The model under review builds one solid part; all positions refer to its coordinate system, in mm. A direction names the side the tool comes from. Coordinates: 2 decimals unless noted, no trailing zeros. Order: outer loops, then holes, each group sorted by start corner. A loop starts at its lowest first (then second) coordinate and runs counter-clockwise, first axis right, second up.
```python
from build123d import *

# Parameters (mm, degrees)
SKETCH_W        = 75.4
SKETCH_H        = 100
PAD_DEPTH       = 16.6
SKETCH005_W     = 71.4
SKETCH005_H     = 96
POCKET_DEPTH    = 14.6
SKETCH006_W     = 21.6
SKETCH006_H     = 11.8
POCKET001_DEPTH = 2
SKETCH007_W     = 21.6
SKETCH007_H     = 11.8
POCKET002_DEPTH = 2
SKETCH008_W     = 7.6
SKETCH008_H     = 8.2
POCKET003_DEPTH = 2
POCKET004_DEPTH = 2
SKETCH010_R     = 3.9
SKETCH010_W     = 16
SKETCH010_H     = 26.5
POCKET005_DEPTH = 2
POCKET005_TAPER = 45
SKETCH011_W     = 15
SKETCH011_H     = 2
PAD005_DEPTH    = 14.6
SKETCH012_R     = 1.1
PAD006_DEPTH    = 8.6
SKETCH013_R     = 1.1
PAD007_DEPTH    = 10.4
FILLET_R        = 2
FILLET001_R     = 4
FILLET002_R     = 1
FILLET003_R     = 6
FILLET004_R     = 5.5
FILLET005_R     = 4
SKETCH022_W     = 31.2
SKETCH022_H     = 29
SKETCH022_W_2   = 28.8
SKETCH022_H_2   = 26.6
PAD013_DEPTH    = 3.4
FILLET011_R     = 8


with BuildPart() as part:
    # Sketch → Pad (new body)
    with BuildSketch(Plane.XY):
        with Locations((0, -28.5)):
            Rectangle(SKETCH_W, SKETCH_H)
    extrude(amount=PAD_DEPTH)

    # Sketch005 (on Face5 of Pad) → Pocket (cut)
    with BuildSketch(Plane(origin=(0, 0, 0), x_dir=(1, 0, 0), z_dir=(0, 0, -1))):
        with Locations((0, 28.5)):
            Rectangle(SKETCH005_W, SKETCH005_H)
    extrude(amount=-POCKET_DEPTH, mode=Mode.SUBTRACT)

    # Sketch006 (on Face3 of Pocket) → Pocket001 (cut)
    with BuildSketch(Plane.YZ.offset(37.7)):
        with Locations((0, 5.9)):
            Rectangle(SKETCH006_W, SKETCH006_H)
    extrude(amount=-POCKET001_DEPTH, mode=Mode.SUBTRACT)

    # Sketch007 (on Face2 of Pocket) → Pocket002 (cut)
    with BuildSketch(Plane(origin=(-37.7, 0, 0), x_dir=(0, -1, 0), z_dir=(-1, 0, 0))):
        with Locations((0, 5.9)):
            Rectangle(SKETCH007_W, SKETCH007_H)
    extrude(amount=-POCKET002_DEPTH, mode=Mode.SUBTRACT)

    # Sketch008 (on Face1 of Pocket) → Pocket003 (cut)
    with BuildSketch(Plane(origin=(0, 21.5, 0), x_dir=(-1, 0, 0), z_dir=(0, 1, 0))):
        with Locations((22, 4.1)):
            Rectangle(SKETCH008_W, SKETCH008_H)
    extrude(amount=-POCKET003_DEPTH, mode=Mode.SUBTRACT)

    # Sketch009 (on Face5 of Pocket) → Pocket004 (cut)
    with BuildSketch(Plane.XY.offset(16.6)):
        with BuildLine():
            Line((15.825713, -15.337742), (15.825713, -16.321696))
            ThreePointArc((15.825713, -16.321696), (16.397859, -17.902616), (17.897046, -18.663599))
            Line((17.897046, -18.663599), (25.282393, -18.663599))
            ThreePointArc((25.282393, -18.663599), (26.185781, -18.272491), (26.544973, -17.355945))
            Line((26.544973, -14.219638), (26.544973, -17.355945))
            ThreePointArc((26.544973, -14.219638), (26.159832, -13.349897), (25.274241, -13.00275))
            Line((17.921865, -13.00275), (25.274241, -13.00275))
            ThreePointArc((17.921865, -13.00275), (16.411472, -13.755218), (15.825713, -15.337742))
        make_face()
    extrude(amount=-POCKET004_DEPTH, mode=Mode.SUBTRACT)

    # Sketch010 (on Face5 of Pocket) → Pocket005 (cut)
    with BuildSketch(Plane.XY.offset(16.6)):
        with Locations((-17.145816, -1.900756)):
            Circle(SKETCH010_R)
        with Locations((10, 2.4)):
            Rectangle(SKETCH010_W, SKETCH010_H)
    extrude(amount=-POCKET005_DEPTH, taper=POCKET005_TAPER, mode=Mode.SUBTRACT)

    # Sketch011 (on Face11 of Pocket) → Pad005 (join)
    with BuildSketch(Plane(origin=(0, 0, 14.6), x_dir=(1, 0, 0), z_dir=(0, 0, -1))):
        with Locations((-28.2, 47.5)):
            Rectangle(SKETCH011_W, SKETCH011_H)
        with Locations((-28.2, 20.5)):
            Rectangle(SKETCH011_W, SKETCH011_H)
        with Locations((28.2, 47.5)):
            Rectangle(SKETCH011_W, SKETCH011_H)
        with Locations((28.2, 20.5)):
            Rectangle(SKETCH011_W, SKETCH011_H)
    extrude(amount=PAD005_DEPTH)

    # Sketch012 (on Face11 of Pocket) → Pad006 (join)
    with BuildSketch(Plane(origin=(0, 0, 14.6), x_dir=(1, 0, 0), z_dir=(0, 0, -1))):
        with BuildLine():
            Line((-35.7, -12.5), (-31.85, -12.5))
            ThreePointArc((-28.85, -15.5), (-29.72868, -13.37868), (-31.85, -12.5))
            Line((-28.85, -19.5), (-28.85, -15.5))
            Line((-28.85, -19.5), (-35.7, -19.5))
            Line((-35.7, -12.5), (-35.7, -19.5))
        make_face()
        with Locations((-31.85, -15.5)):
            Circle(SKETCH012_R, mode=Mode.SUBTRACT)
        with BuildLine():
            Line((28.85, -19.5), (28.85, -15.5))
            ThreePointArc((31.85, -12.5), (29.72868, -13.37868), (28.85, -15.5))
            Line((35.7, -12.5), (31.85, -12.5))
            Line((35.7, -12.5), (35.7, -19.5))
            Line((28.85, -19.5), (35.7, -19.5))
        make_face()
        with Locations((31.85, -15.5)):
            Circle(SKETCH012_R, mode=Mode.SUBTRACT)
        with BuildLine():
            Line((-35.7, 12.5), (-35.7, 19.5))
            Line((-35.7, 19.5), (-28.85, 19.5))
            Line((-28.85, 19.5), (-28.85, 15.5))
            ThreePointArc((-31.85, 12.5), (-29.72868, 13.37868), (-28.85, 15.5))
            Line((-35.7, 12.5), (-31.85, 12.5))
        make_face()
        with Locations((-31.85, 15.5)):
            Circle(SKETCH012_R, mode=Mode.SUBTRACT)
        with BuildLine():
            Line((31.85, 12.5), (35.7, 12.5))
            Line((35.7, 12.5), (35.7, 19.5))
            Line((35.7, 19.5), (28.85, 19.5))
            Line((28.85, 19.5), (28.85, 15.5))
            ThreePointArc((28.85, 15.5), (29.72868, 13.37868), (31.85, 12.5))
        make_face()
        with Locations((31.85, 15.5)):
            Circle(SKETCH012_R, mode=Mode.SUBTRACT)
    extrude(amount=PAD006_DEPTH)

    # Sketch013 (on Face11 of Pocket) → Pad007 (join)
    with BuildSketch(Plane(origin=(0, 0, 14.6), x_dir=(1, 0, 0), z_dir=(0, 0, -1))):
        with BuildLine():
            Line((-35.7, 76.5), (-29.35, 76.5))
            Line((-29.35, 76.5), (-29.35, 72.5))
            ThreePointArc((-31.85, 70), (-30.082233, 70.732233), (-29.35, 72.5))
            Line((-35.7, 70), (-31.85, 70))
            Line((-35.7, 76.5), (-35.7, 70))
        make_face()
        with Locations((-31.85, 72.5)):
            Circle(SKETCH013_R, mode=Mode.SUBTRACT)
        with BuildLine():
            Line((35.7, 76.5), (35.7, 70))
            Line((35.7, 70), (31.85, 70))
            ThreePointArc((29.35, 72.5), (30.082233, 70.732233), (31.85, 70))
            Line((29.35, 76.5), (29.35, 72.5))
            Line((35.7, 76.5), (29.35, 76.5))
        make_face()
        with Locations((31.85, 72.5)):
            Circle(SKETCH013_R, mode=Mode.SUBTRACT)
    extrude(amount=PAD007_DEPTH)

    # Fillet
    fillet_edges = [part.edges().sort_by_distance(p)[0] for p in [
        (-35.7, 0, 14.6),
        (-35.7, -34, 14.6),
        (-35.7, -59.25, 14.6),
        (35.7, 0, 14.6),
        (35.7, -34, 14.6),
        (35.7, -59.25, 14.6),
    ]]
    fillet(fillet_edges, radius=FILLET_R)

    # Fillet001
    fillet001_edges = [part.edges().sort_by_distance(p)[0] for p in [
        (0, 19.5, 14.6),
        (0, -76.5, 14.6),
    ]]
    fillet(fillet001_edges, radius=FILLET001_R)

    # Fillet002
    fillet002_edges = [part.edges().sort_by_distance(p)[0] for p in [
        (-35.7, 19.5, 3),
        (35.7, 19.5, 3),
    ]]
    fillet(fillet002_edges, radius=FILLET002_R)

    # Fillet003
    fillet003_edges = [part.edges().sort_by_distance(p)[0] for p in [
        (-35.7, -76.5, 2.1),
        (35.7, -76.5, 2.1),
    ]]
    fillet(fillet003_edges, radius=FILLET003_R)

    # Fillet004
    fillet004_edges = [part.edges().sort_by_distance(p)[0] for p in [
        (0, 21.5, 16.6),
    ]]
    fillet(fillet004_edges, radius=FILLET004_R)

    # Fillet005
    fillet005_edges = [part.edges().sort_by_distance(p)[0] for p in [
        (37.7, -31.25, 16.6),
        (37.7, 21.5, 5.55),
        (-37.7, -31.25, 16.6),
        (-37.7, 21.5, 5.55),
    ]]
    fillet(fillet005_edges, radius=FILLET005_R)

    # Sketch022 (on Face36 of Pad007) → Pad013 (join)
    with BuildSketch(Plane(origin=(0, 0, 14.6), x_dir=(1, 0, 0), z_dir=(0, 0, -1))):
        with Locations((8.156075, -2.412758)):
            Rectangle(SKETCH022_W, SKETCH022_H)
        with Locations((8.156075, -2.412758)):
            Rectangle(SKETCH022_W_2, SKETCH022_H_2, mode=Mode.SUBTRACT)
    extrude(amount=PAD013_DEPTH)

    # Fillet011
    fillet011_edges = [part.edges().sort_by_distance(p)[0] for p in [
        (0, -78.5, 16.6),
        (37.7, -78.5, 6.3),
        (-37.7, -78.5, 6.3),
    ]]
    fillet(fillet011_edges, radius=FILLET011_R)


with BuildPart() as part_1:
    # Body placement: moved
    add(part.part.moved(Location((0, 0, -2))))


solid = part_1.part
```
(1) Machinability: for faces 4 (the face through (33, -73, 2.2)), 5 (the face through (37, 0, 9.8)), 6 (the face through (22, -13.003, 14)), which of the approach directions +Z, -Z, +X, -X, +Y, -Y give a long, thin tool a straight path to every point of the face, cutting with its end or side? Answer none if there is none.
A:
face 4: -Z
face 5: -Z, +X
face 6: +Z, -Z
(2) For pin 1 Ø1 at (x, y) = (36.5, 5) entering from -Z; pin 2 Ø3.5 at (x, z) = (7, 10) entering from -Y; pin 3 Ø1.5 at (x, z) = (-21.5, 12.5) entering from +Y, all flat-tipped, find the tip position at first contact; note any pin that passes through.
A:
pin 1: stops at z = 9.8
pin 2: stops at y = -78.33
pin 3: stops at y = 20.82
(3) We need section C-C, the plane z = -0.25. Count the separate pieces of the cut face and the enclosed holes in it, and give its area (3 significant figures).
A:
separate pieces: 3
enclosed holes: 0
area: 686 mm2
(4) Wall thickness on probe 1 along X at (y, z) = (-15.5, 8); probe 2 along Y at (x, z) = (25, 4.5): over which ranges is each line inside the solid? List them lowest first.
A:
probe 1: x = -37.7 to -32.95, -30.75 to -28.85, 28.85 to 30.75, 32.95 to 37.7
probe 2: y = -78.5 to -76.5, -48.5 to -46.5, -21.5 to -19.5, 19.5 to 21.5
(5) We need section B-B, the plane x = -22.5. Write out the cut boundary in (y, z).
A:
outline: (-78.5, -2) - (-76.5, -2) - (-76.5, 8.6) arc R4 cw to (-72.5, 12.6) - (-48.5, 12.6) - (-48.5, -2) - (-46.5, -2) - (-46.5, 12.6) - (-21.5, 12.6) - (-21.5, -2) - (-19.5, -2) - (-19.5, 12.6) - (15.5, 12.6) arc R4 cw to (19.5, 8.6) - (19.5, 6.2) - (21.5, 6.2) - (21.5, 9.1) arc R5.5 ccw to (16, 14.6) - (-70.5, 14.6) arc R8 ccw to (-78.5, 6.6) - close
(6) We need section A-A, the plane y = -32. Write out the cut boundary in (x, z).
A:
outline: (-37.7, -2) - (-35.7, -2) - (-35.7, 10.6) arc R2 cw to (-33.7, 12.6) - (33.7, 12.6) arc R2 cw to (35.7, 10.6) - (35.7, -2) - (37.7, -2) - (37.7, 10.6) arc R4 ccw to (33.7, 14.6) - (-33.7, 14.6) arc R4 ccw to (-37.7, 10.6) - close
(7) Draft analysis for pull direction Y (two halves, no side actions). For faces 1 (the face through (-36.497, 20.359, 3.472)), 2 (the face through (37.7, -37, 4)), 3 (the face through (-33, -73, 2.2)), state which applies: released by +Y, released by -Y, zero draft, split by the parting line, or undercut.
A:
face 1: released by +Y
face 2: zero draft
face 3: undercut
